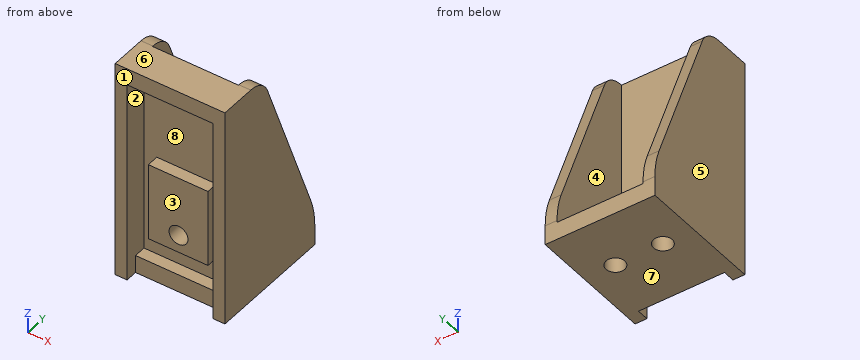
Autodesk Fusion 360 part; units mm, degrees
sketch "vertical plane" plane through (0, 0, 0) normal (0, 1, 0) x (-1, 0, 0)
  circle A0 centre (0, 10) radius 1.6
  line L0 (-7.25, 0) -> (7.25, 0)
  line L1 (7.25, 0) -> (7.25, 37.31)
  line L2 (7.25, 37.31) -> (-7.25, 37.31)
  line L3 (-7.25, 37.31) -> (-7.25, 0)
  line L4 (0, 0) -> (0, 37.31)
  line L5 (-9.25, 0) -> (9.25, 0)
  line L6 (9.25, 0) -> (9.25, 37.3146)
  line L7 (9.25, 37.3146) -> (-9.25, 37.3146)
  line L8 (-9.25, 37.3146) -> (-9.25, 0)
  line L9 (-9.25, 3) -> (9.25, 3)
  line L10 (-7.25, 34.5) -> (7.25, 34.5)
  line L11 (-4.9614, 7) -> (5.0877, 7)
  line L12 (5.0877, 7) -> (5.0877, 20.0804)
  line L13 (5.0877, 20.0804) -> (-4.9614, 20.0804)
  line L14 (-4.9614, 20.0804) -> (-4.9614, 7)
  dimension "d43" = 3.2
  dimension "d72" = 14.5
  dimension "d73" = 2
  dimension "d74" = 3
  dimension "d75" = 31.5
  dimension "d76" = 7
  dimension "d77" = 4
sketch "Sketch25" plane through (0, 0, 0) normal (0, 0, 1) x (1, 0, 0)
  line L0 (9.25, 0) -> (-9.25, 0)
  line L1 (9.25, 0) -> (9.25, 21.23)
  line L2 (9.25, 21.23) -> (-9.25, 21.23)
  line L3 (-9.25, 21.23) -> (-9.25, 0)
  line L4 (-9.25, 12) -> (9.25, 12)
  line L5 (0, 21.23) -> (0, 0)
  line L6 (9.25, 0) -> (-9.25, 0)
  circle A0 centre (-4, 12) radius 1.575
  circle A1 centre (4, 12) radius 1.575
  point P0 (7.25, 0)
  point P1 (9.25, 0)
  point P2 (-7.25, 0)
  point P3 (-9.25, 0)
  dimension "d112" = 21.23
  dimension "d113" = 12
  dimension "d114" = 3.15
  dimension "d115" = 3.15
  dimension "d116" = 8
ref_plane "WorkPlane2" through (9.25, 0, 18.6573) normal (-1, 0, 0) x (0, 0, -1)
sketch "side plane details" plane through (9.25, 0, 0) normal (-1, 0, 0) x (0, -1, 0)
  line L0 (0, 0) -> (-21.2275, 0)
  line L1 (-21.2275, 0) -> (-21.2275, 3)
  line L2 (-21.2275, 3) -> (0, 3)
  line L3 (0, 3) -> (0, 0)
  line L4 (0, 37.3146) -> (-9, 37.3146)
  line L5 (-9, 37.3146) -> (-9, 0)
  line L6 (-9, 0) -> (0, 0)
  line L7 (0, 0) -> (0, 37.3146)
  line L8 (-6, 0) -> (-6, 37.3146)
  line L9 (0, 3) -> (-21.4, 3)
  line L10 (0, 5.7) -> (0, 3)
  line L11 (-21.23, 0) -> (0, 0)
  line L12 (0, 0) -> (0, 5.9996)
  line L13 (0, 5.9996) -> (-21.23, 5.9996)
  line L14 (-21.23, 5.9996) -> (-21.23, 0)
  line L15 (-9, 37.3146) -> (-21.23, 5.9996)
  point P0 (0, 37.3146)
  point P1 (-21.23, 0)
  dimension "d83" = 9
  dimension "d84" = 3
  dimension "d89" = 6
extrude "Extrude25" add sketch "Sketch25" along normal blind 3
extrude "Extrude26" add sketch "vertical plane" along normal blind 6
extrude "Extrude27" cut sketch "vertical plane" along normal blind 2 contours L0 L1 L4 L5 L9 | L0 L3 L4 L5 L9
extrude "Extrude28" cut sketch "vertical plane" along normal blind 4 contours A0 L4 | A0 L4 L11 L12 L13 | A0 L4 | A0 L4 L11 L13 L14 | L3 L4 L9 L10 L11 L13 L14 | L1 L4 L9 L10 L11 L12 L13
extrude "Extrude29" cut sketch "vertical plane" along normal blind 2 from surface at 4 contours A0 L4 | A0 L4
extrude "Extrude30" add sketch "vertical plane" against normal blind 2 from surface at 4 contours A0 L4 L11 L12 L13 | A0 L4 L11 L13 L14
extrude "Extrude31" cut sketch "Sketch25" along normal blind 3 contours L4 A1 | L4 A1 | L4 A0 | L4 A0
extrude "Extrude32" add sketch "side plane details" along normal blind 2 contours L2 L5 L8 L9 L13 | L2 L5 L9 L13 L14 | L4 L5 L8 L13 | L5 L13 L15
extrude "Extrude33" add 1 faces at (7.25, 12.0767, 15.4381) along direction (-1, 0, 0) blind 2 from surface at 14.5
fillet "Fillet1" radius 4.25 2 edges at (8.25, 9, 37.3146) (-8.25, 9, 37.3146)
fillet "Fillet2" radius 14.25 2 edges at (-8.25, 21.23, 5.9996) (8.25, 21.23, 5.9996)
Read the model definition and answer for the solid it produces. Units are mm, in the model's axes. Face numbers are marked on the shaded views. A direction names the side the tool comes from. Coordinates: 2 decimals unless noted, no trailing zeros. Write each loop counter-clockwise with the first axis right and the second up, starting at its lowest first coordinate (ties: lowest second). Pieces come first, ordered by that corner, then holes. Notation, with made-up numbers: (37.25, 6.5) -> (73.25, 6.5) arc R18 cw to (73.25, 20.5) -> close; hole circle Ø5 at (77.25, 70.5). An arc over 180 degrees is marked (long way). Write item = value, one per line.
(1) Which of the six approach directions +Z, -Z, +X, -X, +Y, -Y give full straight-line access (tool end or side, diameter ignored) to the marked faces 1, 2, 3 and 4?
From the geometry:
face_1 = +Z, -Z, +X, -X, -Y
face_2 = -Y
face_3 = -Z, -Y
face_4 = +Z, +Y
(2) For a pull along Z with two mould halves and no side action, classify the marked faces 5, 6, 7 and 8 as +Z half, -Z half, draft (parallel to the pull), parting line (faces both ways), or undercut.
From the geometry:
face_5 = draft
face_6 = +Z half
face_7 = -Z half
face_8 = undercut
(3) Section A-A on y = 3.25 is taken. Write down the section's boundary in (x, z).
From the geometry:
outline = (-9.25, 0) -> (9.25, 0) -> (9.25, 37.31) -> (-9.25, 37.31) -> close; (-5.09, 7) -> (4.96, 7) -> (4.96, 20.08) -> (-5.09, 20.08) -> close; hole (-7.25, 3) -> (7.25, 3) -> (7.25, 34.5) -> (-7.25, 34.5) -> close; hole circle Ø3.2 at (0, 10)
(4) Section C-C on z = 10 is taken. Write down the section's boundary in (x, y).
From the geometry:
outline = (-9.25, 0) -> (-7.25, 0) -> (-7.25, 4) -> (-5.09, 4) -> (-5.09, 2) -> (-1.6, 2) -> (-1.6, 6) -> (-7.25, 6) -> (-7.25, 19.67) -> (-9.25, 19.67) -> close; (1.6, 2) -> (4.96, 2) -> (4.96, 4) -> (7.25, 4) -> (7.25, 0) -> (9.25, 0) -> (9.25, 19.67) -> (7.25, 19.67) -> (7.25, 6) -> (1.6, 6) -> close
(5) Section B-B on x = 4 is taken. Write down the section's boundary in (y, z) (3 decimals).
From the geometry:
outline = (0, 34.5) -> (4, 34.5) -> (4, 20.08) -> (2, 20.08) -> (2, 7) -> (4, 7) -> (4, 3) -> (2, 3) -> (2, 0) -> (10.425, 0) -> (10.425, 3) -> (6, 3) -> (6, 37.315) -> (0, 37.315) -> close; (13.575, 0) -> (21.23, 0) -> (21.23, 3) -> (13.575, 3) -> close
(6) Straight lines are drawn through the part: L1, parallel to X at y = 12, z = 0.8 (3 decimals); L2, parallel to Z at x = 0, y = 3.7; L3, parallel to X at y = 6.75, z = 21. For each, find the intervals that lie inside material, in ascending order. Write a range as from..to.
From the geometry:
L1 = -9.25..-5.575, -2.425..2.425, 5.575..9.25
L2 = 0..3, 7..8.4, 11.6..20.08, 34.5..37.31
L3 = -9.25..-7.25, 7.25..9.25
(7) Given pin 1 Ø7 at (x, z) = (1.5, 24) entering from -Y; pin 2 Ø3 at (x, z) = (-1, 12.5) entering from -Y; pin 3 Ø1.5 at (x, y) = (5.5, 10.5) entering from +Z, each flat-ended and moving along its own axis, determine where each tip first touches the part or whether it passes through.
From the geometry:
pin_1 = 4
pin_2 = 2
pin_3 = 3
(8) Section D-D on x = 6.75 is taken. Write down the section's boundary in (y, z).
From the geometry:
outline = (0, 34.5) -> (4, 34.5) -> (4, 3) -> (2, 3) -> (2, 0) -> (21.23, 0) -> (21.23, 3) -> (6, 3) -> (6, 37.31) -> (0, 37.31) -> close
